Could you check a few things on this model? Use its own coordinates, in mm. A direction names the side the tool comes from. Coordinates: 2 decimals unless noted, no trailing zeros. Order: outer loops, then holes, each group sorted by start corner. A loop starts at its lowest first (then second) coordinate and runs counter-clockwise, first axis right, second up. Notation, with made-up numbers: M 29.25,10 L 53.25,10 A14 ccw 53.25,26 Z; hole C 4,-10 d11. An arc over 180 degrees is marked long. Write item = value, one per line. Start each with the question number.
from build123d import *

# Parameters (mm, degrees)
SKETCH2_W           = 20
SKETCH2_H           = 100
BOSS_EXTRUDE1_DEPTH = 10
SKETCH3_R           = 3.9
BOSS_EXTRUDE2_DEPTH = 12
BOSS_EXTRUDE3_DEPTH = 1
SKETCH5_R           = 3.9
BOSS_EXTRUDE4_DEPTH = 7
SKETCH6_W           = 20
SKETCH6_H           = 2
CUT_EXTRUDE1_DEPTH  = 9


with BuildPart() as part:
    # Sketch2 → Boss-Extrude1 (new body)
    with BuildSketch(Plane.XY):
        with Locations((-42.577319588, 46.391752577)):
            Rectangle(SKETCH2_W, SKETCH2_H)
    extrude(amount=BOSS_EXTRUDE1_DEPTH)

    # Sketch3 → Boss-Extrude2 (add)
    with BuildSketch(Plane.XZ.offset(3.608247423)):
        with Locations(Location((-42.577319588, 5, 0), (0, 0, 270))):
            Circle(SKETCH3_R)
    extrude(amount=BOSS_EXTRUDE2_DEPTH)

    # Sketch4 → Boss-Extrude3 (add)
    with BuildSketch(Plane.XY.offset(10)):
        with BuildLine():
            Line((-32.577319588, 96.391752577), (-32.577319588, 101.758502997))
            ThreePointArc((-32.577319588, 101.758502997), (-42.577319588, 120.391752577), (-52.577319588, 101.758502997))
            Line((-52.577319588, 101.758502997), (-52.577319588, 96.391752577))
            Line((-52.577319588, 96.391752577), (-32.577319588, 96.391752577))
        make_face()
    extrude(amount=-BOSS_EXTRUDE3_DEPTH)

    # Sketch5 → Boss-Extrude4 (add)
    with BuildSketch(Plane(origin=(0, 0, 9), x_dir=(-1, 0, 0), z_dir=(0, 0, -1))):
        with Locations(Location((42.577319588, 108.391752577, 0), (0, 0, 180))):
            Circle(SKETCH5_R)
    extrude(amount=BOSS_EXTRUDE4_DEPTH)

    # Sketch6 → Cut-Extrude1 (cut)
    with BuildSketch(Plane(origin=(0, 0, 0), x_dir=(-1, 0, 0), z_dir=(0, 0, -1))):
        with Locations((42.577319588, 95.391752577)):
            Rectangle(SKETCH6_W, SKETCH6_H)
    extrude(amount=-CUT_EXTRUDE1_DEPTH, mode=Mode.SUBTRACT)


solid = part.part
(1) Imagine slicing it at B-B on y = 99. List the corners of the cut face in (x, z) for me, plus the area to 3 significant figures.
(2) Please list where these lines run through material, in increasing order: probe 1 along Y at (x, z) = (-42.5, 5.75); probe 2 along Y at (x, z) = (-52.25, 0.75); probe 3 along X at (y, z) = (41.5, 2.25). Write a range as from..to.
(3) Imagine slicing it at D-D on y = 5. List the corners of the cut face in (x, z) for me, plus the area to 3 significant figures.
(4) For faces 1 (the flat face through (-43, 108, 2)), 2 (the cylindrical face through (-40.778, 111.852, 5.549)), 3 (the flat face through (-52.577, 50, 5)), 4 (the cylindrical face through (-38.71, -9.52, 5.51)), 5 (the flat face through (-42, 94.392, 4)), which set-ups out of +Z, -Z, +X, -X, +Y, -Y let a thin tool reach every point of the face, with its end or its side?
(5) Imagine slicing it at C-C on x = -35.25. List the corners of the cut face in (y, z) for me.
(6) Will these pins go through, and if not, where does the flat tip stop? P1, Ø2, axis at x = -36, z = 7.5, coming from the -Y side; P2, Ø3, axis at y = 34.5, z = 3, coming from the -X side; P3, Ø2.5, axis at x = -44.5, z = 6, coming from the +Y side.
(7) Imagine slicing it at A-A on z = 5. List the corners of the cut face in (x, y) for me, plus the area to 3 significant figures.
(8) Thinking about a two-plate mould opening in Y: for faces 6 (the cylindrical face through (-42.215, 120.386, 9.507)), 7 (the flat face through (-40, 105, 9)), 8 (the flat face through (-32.577, 48, 5)), which applies, released by +Y, released by -Y, zero draft, split by the parting line, or undercut?
Response:
q1.outline = M -52.58,9 L -32.58,9 L -32.58,10 L -52.58,10 Z
q1.area = 20.0 mm2
q2.probe_1 = -15.61..94.39, 104.49..112.29
q2.probe_2 = -3.61..94.39
q2.probe_3 = -52.58..-32.58
q3.outline = M -52.58,0 L -32.58,0 L -32.58,10 L -52.58,10 Z
q3.area = 200 mm2
q4.face_1 = -Z, +X, -X, +Y
q4.face_2 = -Z
q4.face_3 = +Z, -Z, -X, -Y
q4.face_4 = -Y
q4.face_5 = -Z, +X, -X
q5.outline = M -3.61,0 L 94.39,0 L 94.39,9 L 117.89,9 L 117.89,10 L -3.61,10 Z
q6.P1 = -3.61
q6.P2 = -52.58
q6.P3 = 112.23
q7.outline = M -52.58,-3.61 L -46.48,-3.61 L -46.48,-15.61 L -38.68,-15.61 L -38.68,-3.61 L -32.58,-3.61 L -32.58,94.39 L -52.58,94.39 Z; C -42.58,108.39 d7.8
q7.area = 2,100 mm2
q8.face_6 = split by the parting line
q8.face_7 = undercut
q8.face_8 = zero draft
